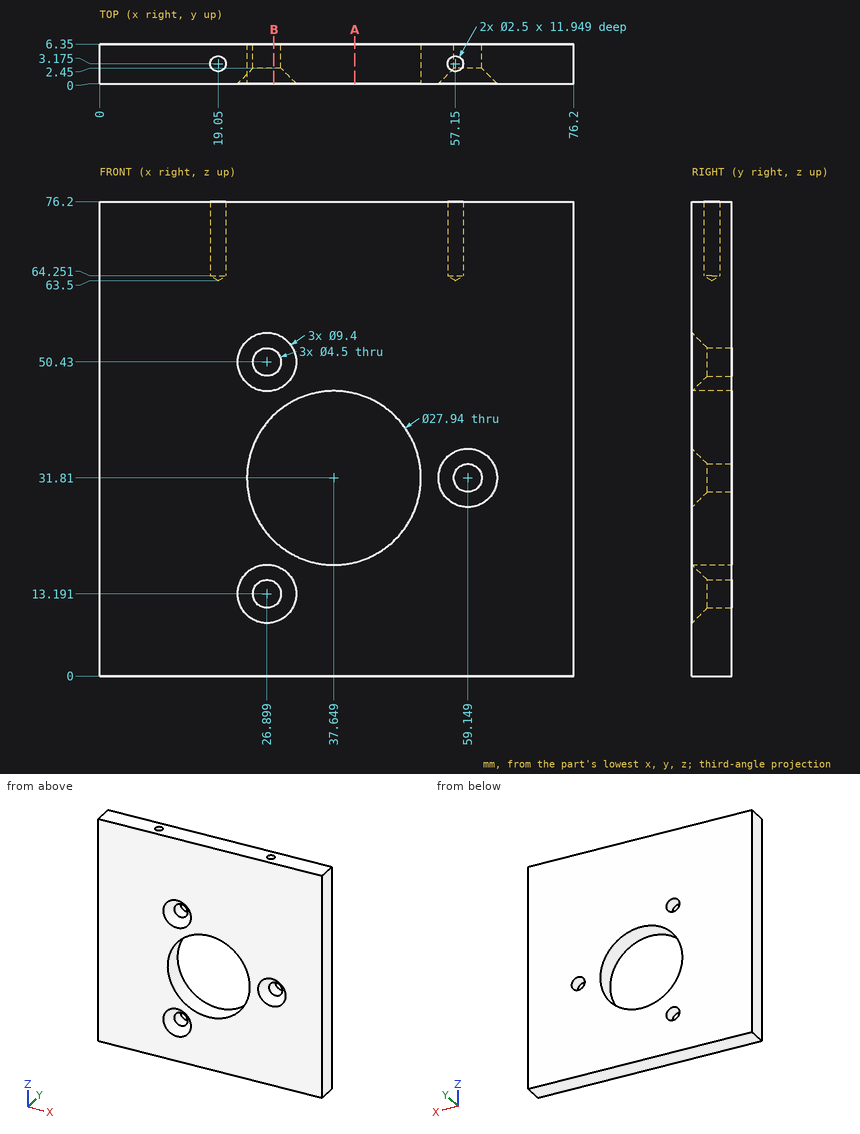
Can you work these out from the drawing? Everything is in mm from the part's minimum corner. Round coordinates to 2 decimals unless told otherwise and drop trailing zeros. Write each loop counter-clockwise with the first axis right and the second up, starting at its lowest first coordinate (ties: lowest second). Pieces come first, ordered by that corner, then holes.
1. Will these pins go through, and if not, where does the flat tip stop? pin 1 Ø5 at (x, z) = (59.15, 31.81) entering from -Y; pin 2 Ø6 at (x, z) = (26.9, 50.43) entering from -Y.
2. Suppose I cut it at A-A (x = 41). List the corners of the cut face in (y, z) for me, and give its area (3 significant figures).
3. I need wall thicknesses on L1, parallel to Z at x = 37.5, y = 2; L2, parallel to X at y = 2, z = 25.5 (1 decimal); L3, parallel to Z at x = 27.5, y = 1.25 (1 decimal). Which ranges of each line are inside material? Lowest first, please.
4. Suppose I cut it at B-B (x = 28). State how many separate pieces and enclosed holes the cut face has, and give its area (3 significant figures).
Answer sheet:
1. pin 1: stops at y = 2.2
1. pin 2: stops at y = 1.7
2. outline: (0, 0) - (6.35, 0) - (6.35, 18.25) - (0, 18.25) - close; (0, 45.37) - (6.35, 45.37) - (6.35, 76.2) - (0, 76.2) - close
2. area: 312 mm2
3. L1: z = 0 to 17.84, 45.78 to 76.2
3. L2: x = 0 to 25.2, 50.1 to 76.2
3. L3: z = 0 to 9.8, 16.6 to 22.2, 41.4 to 47, 53.8 to 76.2
4. separate pieces: 4
4. enclosed holes: 0
4. area: 293 mm2
